Design review of the part shown in the three views and the two pictorial views. Dimensions are in mm from the part's minimum x, y and z. A direction names the side the tool comes from. Round coordinates to 2 decimals unless told otherwise and drop trailing zeros. Write each loop counter-clockwise with the first axis right and the second up, starting at its lowest first coordinate (ties: lowest second). Pieces come first, ordered by that corner, then holes. Notation, with made-up numbers: (46.5, 55.5) -> (67.5, 55.5) arc R23 ccw to (67.5, 79.5) -> close; hole circle Ø10 at (41, -23). An arc over 180 degrees is marked (long way). Answer as a JSON object with one key per item and string values. Group by question number.
1) We need section D-D, the plane y = 2.75. Write out the cut boundary in (x, z).
2) Insertion check: pin 1 Ø2 at (y, z) = (3, 7.5) entering from +X; pin 2 Ø3.5 at (y, z) = (7.75, 2.75) entering from -X; pin 3 Ø6.5 at (y, z) = (2.75, 7.75) entering from -X. Each pin has a flat end and moves straight along its axis. Give the tip position at first contact, or say it passes through.
3) To check wall thickness, follow probe 1 along Z at (x, y) = (9.9, 7.75); probe 2 along Z at (x, y) = (10, 8.5) (1 decimal); probe 3 along Y at (x, z) = (10, 7.75). State the ranges of each line that lie inside material, in increasing order. Write a range as [from, to].
4) We need section C-C, the plane z = 3.5. Write out the cut boundary in (x, y).
5) Machinability: for the marked faces 1, 2 and 3, which of the approach directions +Z, -Z, +X, -X, +Y, -Y give a long, thin tool a straight path to every point of the face, cutting with its end or side? Answer none if there is none.
6) Mouldability with a two-part tool opening along Y and no side actions: class the marked faces 4, 5, 6 and 7 as pulls with the +Y half, pulls with the -Y half, needs draft (parallel to the pull), parting line crosses it, or undercut.
7) We need section A-A, the plane y = 7.75. Count the separate pieces of the cut face and the enclosed holes in it.
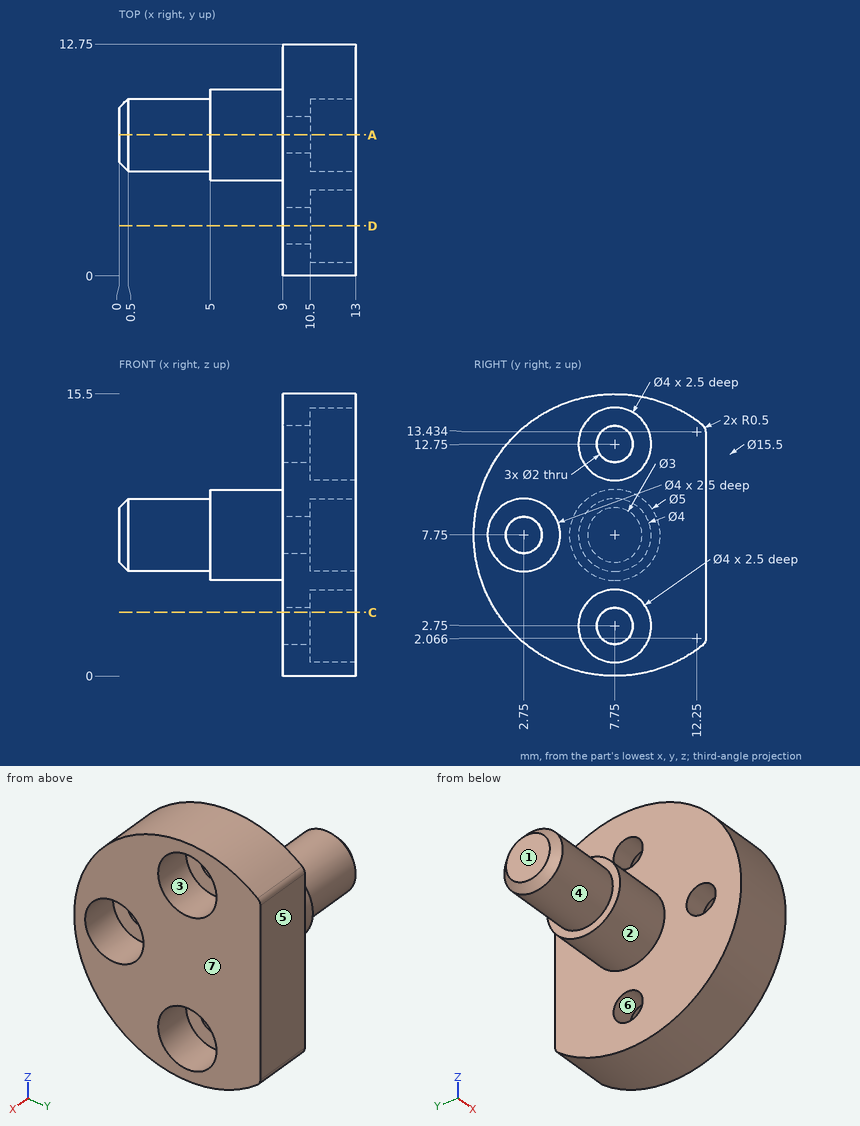
Here are the results:
{
 "1": {"outline": "(9, 1.83) -> (13, 1.83) -> (13, 5.75) -> (10.5, 5.75) -> (10.5, 6.75) -> (9, 6.75) -> close; (9, 8.75) -> (10.5, 8.75) -> (10.5, 9.75) -> (13, 9.75) -> (13, 13.67) -> (9, 13.67) -> close"},
 "2": {"pin 1": "stops at x = 10.5", "pin 2": "stops at x = 9", "pin 3": "stops at x = 0.25"},
 "3": {"probe 1": "z = [0, 1.75], [3.75, 11.75], [13.75, 15.5]", "probe 2": "z = [0, 2.1], [3.4, 12.1], [13.4, 15.5]", "probe 3": "y = [0, 1.75], [3.75, 12.75]"},
 "4": {"outline": "(9, 1.27) -> (13, 1.27) -> (13, 5.9) -> (10.5, 5.9) -> (10.5, 7.09) -> (9, 7.09) -> close; (9, 8.41) -> (10.5, 8.41) -> (10.5, 9.6) -> (13, 9.6) -> (13, 12.75) -> (9, 12.75) -> close"},
 "5": {"face 1": "+Z, -Z, -X, +Y, -Y", "face 2": "-X", "face 3": "+X"},
 "6": {"face 4": "parting line crosses it", "face 5": "pulls with the +Y half", "face 6": "undercut", "face 7": "needs draft"},
 "7": {"separate pieces": "3", "enclosed holes": "0"}
}
